CAD build for the part. Positions are in the model's coordinates, mm. A direction names the side the tool comes from. Round coordinates to 2 decimals unless told otherwise and drop trailing zeros. Loops run counter-clockwise (first coordinate to the right, second up) from the corner with the lowest first, then second, coordinate; pieces in that order, holes last. Notation, with made-up numbers: M 63,20 L 122,20 A21 ccw 122,58 Z; hole C 33.5,-16 d1. An arc over 180 degrees is marked long. Use a Markdown table: item, result. Add a question column.
(1) Wall check: L1, parallel to Y at x = 0.2, z = 19; L2, parallel to Z at x = 2.4, y = 1.1; L3, parallel to X at y = -0.25, z = 11. Give the ranges that are in metal, low to high.
(2) Band-saw the part on B-B, the plane z = -33. Write the cut outline in (x, y), and give its area (3 significant figures).
(3) Which spindle directions (+Z, -Z, +X, -X, +Y, -Y) get a long thin tool onto all of the face, cutting with end or side? Do faces 1 (the face through (-1.9, -0.08, 22.62)), 2 (the face through (-1.4, -0.06, 39.13)). Say none if no direction does.
(4) Band-saw the part on A-A, the plane z = 36. Write the cut outline in (x, y).
(5) Two-plate mould, pull along Z, no slides. Class faces 3 (the face through (-1.4, -0.06, 48.13)), 4 (the face through (0, 0, 50.117)), 5 (the face through (-1.9, -0.08, 25.62)): released by +Z, released by -Z, zero draft, split by the parting line, or undercut.
(6) Flat gauge pins, fed straight in: P1, Ø1.5, axis at x = 1.5, z = -8, coming from the +Y side; P2, Ø2, axis at y = -2, z = -18.5, coming from the +X side. Where does each tip first touch, or does it go through?
from build123d import *

# Parameters (mm, degrees)
F0_W   = 1
F0_H   = 1
F0_W_2 = 0.5
F0_H_2 = 2


with BuildPart() as f1:
    # F0 (on Front) → F1 (revolve)
    with BuildSketch(Plane.XZ):
        Polygon((1.9, 50.117493), (0, 50.117493), (0, -49.882507), (1.9, -49.882507), (1.9, -48.882507), (1.4, -48.882507), (1.4, -46.882507), (1.9, -46.882507), (1.9, 19.117493), (1.9, 20.117493), (1.4, 20.117493), (1.4, 22.117493), (1.9, 22.117493), (1.9, 23.117493), (1.4, 23.117493), (1.4, 25.117493), (1.9, 25.117493), (1.9, 26.117493), (1.4, 26.117493), (1.4, 28.117493), (1.9, 28.117493), (1.9, 29.117493), (1.4, 29.117493), (1.4, 31.117493), (1.9, 31.117493), (1.9, 32.117493), (1.4, 32.117493), (1.4, 34.117493), (1.9, 34.117493), (1.9, 34.617493), (1.9, 35.117493), (1.4, 35.117493), (1.4, 37.117493), (1.9, 37.117493), (1.9, 38.117493), (1.4, 38.117493), (1.4, 40.117493), (1.9, 40.117493), (1.9, 41.117493), (1.4, 41.117493), (1.4, 43.117493), (1.9, 43.117493), (1.9, 44.117493), (1.4, 44.117493), (1.4, 46.117493), (1.9, 46.117493), (1.9, 47.117493), (1.4, 47.117493), (1.4, 49.117493), (1.9, 49.117493), align=None)
        with Locations((2.4, -49.382507)):
            Rectangle(F0_W, F0_H)
        with Locations((1.65, -47.882507)):
            Rectangle(F0_W_2, F0_H_2)
    revolve(axis=Axis((0, 0, 0.117493), (0, 0, -1)))


solid = f1.part
Return value:
| question | item | result |
|---|---|---|
| 1 | L1 | -1.89 to 1.89 |
| 1 | L2 | -49.88 to -48.88 |
| 1 | L3 | -1.88 to 1.88 |
| 2 | outline | C 0,0 d3.8 |
| 2 | area | 11.3 mm^2 |
| 3 | face 1 | +Z |
| 3 | face 2 | none |
| 4 | outline | C 0,0 d2.8 |
| 5 | face 3 | undercut |
| 5 | face 4 | released by +Z |
| 5 | face 5 | zero draft |
| 6 | P1 | y = 1.75 |
| 6 | P2 | x = 1.62 |
